Drawing for the job (mm, zero at the part's lowest x, y, z). A direction names the side the tool comes from. Give positions to 0.01 mm unless a question says otherwise; leave off trailing zeros. Order: outer loops, then holes, each group sorted by start corner. A loop starts at its lowest first (then second) coordinate and runs counter-clockwise, first axis right, second up. Notation, with made-up numbers: (26.5, 35) - (62.5, 35) arc R25 ccw to (62.5, 57) - close; hole circle Ø11 at (59.5, -27.5). An arc over 180 degrees is marked (long way). One line per item, written item: value.
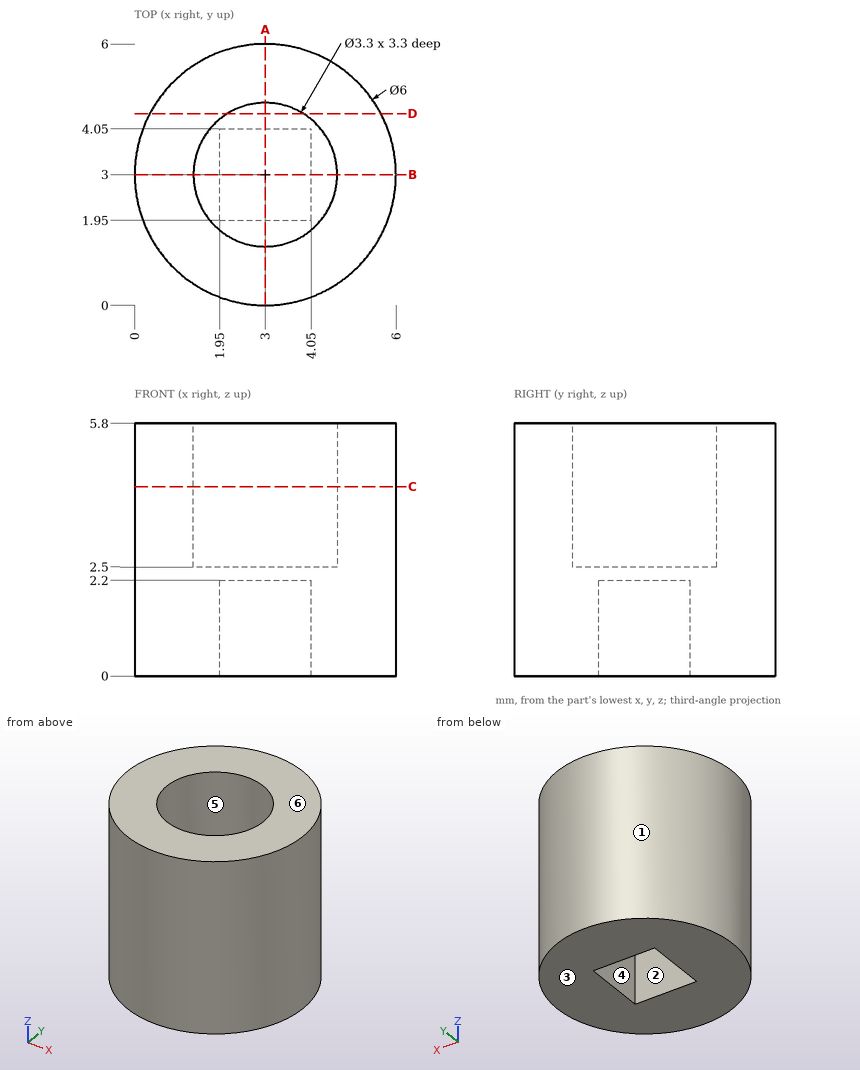
1) Mould opens along Y. For the marked faces 1, 2 and 3 say: released by +Y, released by -Y, zero draft, split by the parting line, or undercut.
Outcome:
face 1: split by the parting line
face 2: undercut
face 3: zero draft
2) Cut at A-A, the plane x = 3. Give the cut face in (y, z), then the cut area to 3 significant figures.
Outcome:
outline: (0, 0) - (1.95, 0) - (1.95, 2.2) - (4.05, 2.2) - (4.05, 0) - (6, 0) - (6, 5.8) - (4.65, 5.8) - (4.65, 2.5) - (1.35, 2.5) - (1.35, 5.8) - (0, 5.8) - close
area: 19.3 mm^2
3) Cut at C-C, the plane z = 4.35. Give the cut face in (x, y).
Outcome:
outline: circle Ø6 at (3, 3); hole circle Ø3.3 at (3, 3)
4) Pin check, flat tips, straight feed: pin 1 (1.5 mm diameter, centred on x = 1, z = 4, fed in from +Y); pin 2 (1.5 mm diameter, centred on y = 1.5, z = 0.5, fed in from -X); pin 3 (1 mm diameter, centred on x = 4, z = 0.5, fed in from -Y). Stop position of each tip, or through.
Outcome:
pin 1: stops at y = 5.73
pin 2: stops at x = 0.1
pin 3: stops at y = 0.04
5) Drill centre lines: line 1 along Y through (x, z) = (3, 3.35); line 2 along Y through (x, z) = (3.1, 0.4); line 3 along Z through (x, y) = (3.05, 2.3). Where is each one in solid material? Low to high. Write a range as from..to.
Outcome:
line 1: y = 0..1.35, 4.65..6
line 2: y = 0..1.95, 4.05..6
line 3: z = 2.2..2.5
6) Cut at D-D, the plane y = 4.4. Give the cut face in (x, z).
Outcome:
outline: (0.35, 0) - (5.65, 0) - (5.65, 5.8) - (3.87, 5.8) - (3.87, 2.5) - (2.13, 2.5) - (2.13, 5.8) - (0.35, 5.8) - close
7) Which spindle directions (+Z, -Z, +X, -X, +Y, -Y) get a long thin tool onto all of the face, cutting with end or side? Do the marked faces 4, 5 and 6. Say none if no direction does.
Outcome:
face 4: -Z
face 5: +Z
face 6: +Z, +X, -X, +Y, -Y
